from build123d import *

# Parameters (mm, degrees)
SKETCH1_W           = 52
SKETCH1_H           = 5.2
BOSS_EXTRUDE1_DEPTH = 8.35
SKETCH2_R           = 0.5
CUT_EXTRUDE1_DEPTH  = 3
SKETCH3_R           = 0.2
BOSS_EXTRUDE2_DEPTH = 12.1
LPATTERN1_COUNT     = 20
LPATTERN1_PITCH     = 2.54


with BuildPart() as part:
    # Sketch1 → Boss-Extrude1 (new body)
    with BuildSketch(Plane(origin=(0, 0, 0), x_dir=(1, 0, 0), z_dir=(0, 1, 0))):
        Rectangle(SKETCH1_W, SKETCH1_H)
    extrude(amount=BOSS_EXTRUDE1_DEPTH)

    # Sketch2 → Cut-Extrude1 (cut)
    with BuildSketch(Plane(origin=(0, 8.35, 0), x_dir=(1, 0, 0), z_dir=(0, 1, 0))):
        with Locations((-24.43, 1.27)):
            Circle(SKETCH2_R)
        with Locations((-24.43, -1.27)):
            Circle(SKETCH2_R)
    cut_extrude1 = extrude(amount=-CUT_EXTRUDE1_DEPTH, mode=Mode.SUBTRACT)

    # Sketch3 → Boss-Extrude2 (add)
    with BuildSketch(Plane.XZ):
        with Locations((-24.43, 1.27)):
            Circle(SKETCH3_R)
        with Locations((-24.43, -1.27)):
            Circle(SKETCH3_R)
    boss_extrude2 = extrude(amount=BOSS_EXTRUDE2_DEPTH)

    # LPattern1: Cut-Extrude1, Boss-Extrude2 ×20
    with Locations(*[(i * LPATTERN1_PITCH, 0, 0) for i in range(1, LPATTERN1_COUNT)]):
        add(cut_extrude1, mode=Mode.SUBTRACT)
        add(boss_extrude2)


solid = part.part
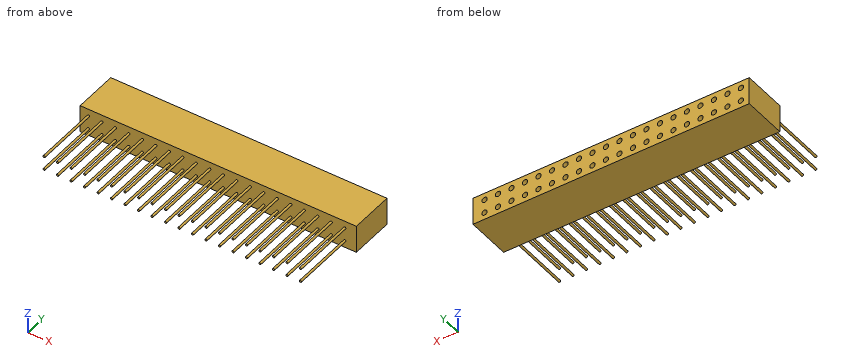
Read the model definition and answer for the solid it produces. Units are mm, in the model's axes. Round coordinates to 2 decimals unless told otherwise and drop trailing zeros. Write each loop counter-clockwise with the first axis right and the second up, starting at its lowest first coordinate (ties: lowest second). Pieces come first, ordered by that corner, then holes.
1. Straight lines are drawn through the part: L1, parallel to Z at x = -6.65, y = 7; L2, parallel to Z at x = -9.5, y = 6; L3, parallel to Y at x = 17.5, z = -2.1. For each, find the intervals that lie inside material, in ascending order.
2. The part is cut by section B-B, the plane x = 15. Determine the outline of the cut face in (y, z).
3. Given pin 1 Ø0.5 at (x, z) = (18.5, 1) entering from +Y; pin 2 Ø6 at (x, y) = (-6.5, -3.5) entering from -Z; pin 3 Ø1 at (y, z) = (-5.5, 1.5) entering from -X, each flat-ended and moving along its own axis, determine where each tip first touches the part or whether it passes through.
4. The part is cut by section A-A, the plane y = -8.25. State how many separate pieces and enclosed holes the cut face has, then the cut area to 3 significant figures.
Values:
1. L1: z = -2.6 to -1.77, -0.77 to 0.77, 1.77 to 2.6
1. L2: z = -2.6 to -1.66, -0.88 to 0.88, 1.66 to 2.6
1. L3: y = 0 to 8.35
2. outline: (0, -2.6) - (8.35, -2.6) - (8.35, 2.6) - (0, 2.6) - close
3. pin 1: stops at y = 8.35
3. pin 2: stops at z = -1.47
3. pin 3: stops at x = -24.63
4. separate pieces: 40
4. enclosed holes: 0
4. area: 5.03 mm2
